Input: part model. Units: mm. Frame: model coordinates. Face numbers are marked on the shaded views. Round coordinates to 2 decimals unless told otherwise and drop trailing zeros. Loops run counter-clockwise (first coordinate to the right, second up) from the corner with the lowest first, then second, coordinate; pieces in that order, holes last. Notation, with made-up numbers: M -31.75,43.5 L -15.75,43.5 A27 cw -15.75,73.5 Z; hole C 69,1.25 d2. An arc over 180 degrees is marked long. Return JSON: item names as keys, results as strings. Group by question number.
1) Section A-A (z = 0). Output: boundary loops of the cut face in (x, y).
2) Section B-B (y = 125). Output: boundary loops of the cut face in (x, z), plus the area to 3 significant figures.
3) Contact query for flat-ended pins moving along their axis: P1, Ø5, axis at x = -17, z = 15.5, coming from the +Y side; P2, Ø22.5, axis at y = -52, z = 3.5, coming from the -X side; P3, Ø8, axis at x = -24.5, z = 19.5, coming from the +Y side. Output: stop coordinate, or through.
4) Mould query, pull axis Z, two halves, no side actions, for the marked faces 1 and 2. Classes: +Z half, -Z half, draft (parallel to the pull), parting line (faces both ways), or undercut.
5) Material intervals for line 1 (Y direction, x = 117, z = -12); line 2 (Z direction, x = 56, y = 189); line 3 (Y direction, x = 114.5, z = -6), sorted ascending. Write a range as from..to.
6) Section C-C (z = -16.5). Output: boundary loops of the cut face in (x, y), plus the area to 3 significant figures.
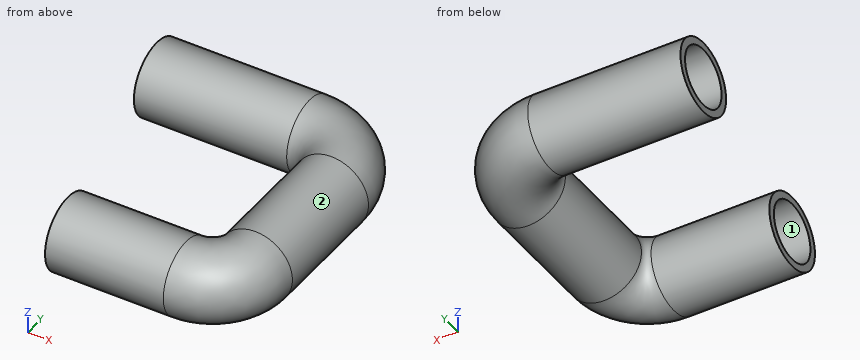
Autodesk Inventor part; units mm, degrees
ref_plane "YZ Plane" through (0, 0, 0) normal (1, 0, 0) x (0, 1, 0)
ref_plane "XZ Plane" through (0, 0, 0) normal (0, 1, 0) x (-1, 0, 0)
ref_plane "XY Plane" through (0, 0, 0) normal (0, 0, 1) x (1, 0, 0)
sketch "Sketch1" plane through (0, 0, 0) normal (1, 0, 0) x (0, 1, 0)
  circle A0 centre (-37.5, 0) radius 37.5
  point P0 (0, 0)
  dimension "d7" = 75
sketch3d "3D Sketch2"
  line L0 (0, -24, 0) -> (120, -24, 0)
  arc A0 (120, -24, 0) -> (150, 6, 0) centre (120, 6, 0) ccw
  line L1 (150, 6, 0) -> (150, 131, 0)
  arc A1 (150, 131, 0) -> (105, 176, 0) centre (105, 131, 0) ccw
  line L2 (105, 176, 0) -> (-50, 176, 0)
  dimension "d0" = 150
  dimension "d1" = 200
  dimension "d2" = 30
  dimension "d3" = 200
  dimension "d4" = 45
sweep "Sweep1" add profiles "Sketch1" path "3D Sketch2"
sketch "Sketch2" plane through (-50, 189.5, 0) normal (-1, 0, 0) x (0, 0, 1)
  circle A0 centre (0, 0) radius 30
  point P0 (0, -189.5)
  dimension "d10" = 60
extrude "Extrusion1" cut sketch "Sketch2" against normal blind 170
sketch "Sketch3" plane through (0, -37.5, 0) normal (-1, 0, 0) x (0, 0, 1)
  circle A0 centre (0, 0) radius 30
  point P0 (0, 37.5)
  dimension "d13" = 60
extrude "Extrusion2" cut sketch "Sketch3" against normal blind 150
properties part number "vacuum"
Returned:
{
 "1": {"outline": "M -50,152 L 105,152 A21 cw 126,131 L 126,6 A6 cw 120,0 L 0,0 L 0,-7.5 L 150,-7.5 L 150,-67.5 L 0,-67.5 L 0,-75 L 120,-75 A81 ccw 201,6 L 201,131 A96 ccw 105,227 L -50,227 L -50,219.5 L 120,219.5 L 120,159.5 L -50,159.5 Z"},
 "2": {"outline": "C 163.5,0 d75", "area": "4,420 mm^2"},
 "3": {"P1": "stops at y = 224.67", "P2": "stops at x = 150", "P3": "stops at y = 223.65"},
 "4": {"face 1": "undercut", "face 2": "parting line"},
 "5": {"line 1": "y = -73.03..-65, -10..-1.97, 150.59..162, 217..224.26", "line 2": "z = -37.5..-30, 30..37.5", "line 3": "y = -74.52..-66.89, -8.11..-0.48, 150.27..160.11, 218.89..226.04"},
 "6": {"outline": "M -50,155.83 L 105,155.83 A24.83 cw 129.83,131 L 129.83,6 A9.83 cw 120,-3.83 L 0,-3.83 L 0,-12.45 L 150,-12.45 L 150,-62.55 L 0,-62.55 L 0,-71.17 L 120,-71.17 A77.17 ccw 197.17,6 L 197.17,131 A92.17 ccw 105,223.17 L -50,223.17 L -50,214.55 L 120,214.55 L 120,164.45 L -50,164.45 Z", "area": "21,700 mm^2"}
}
